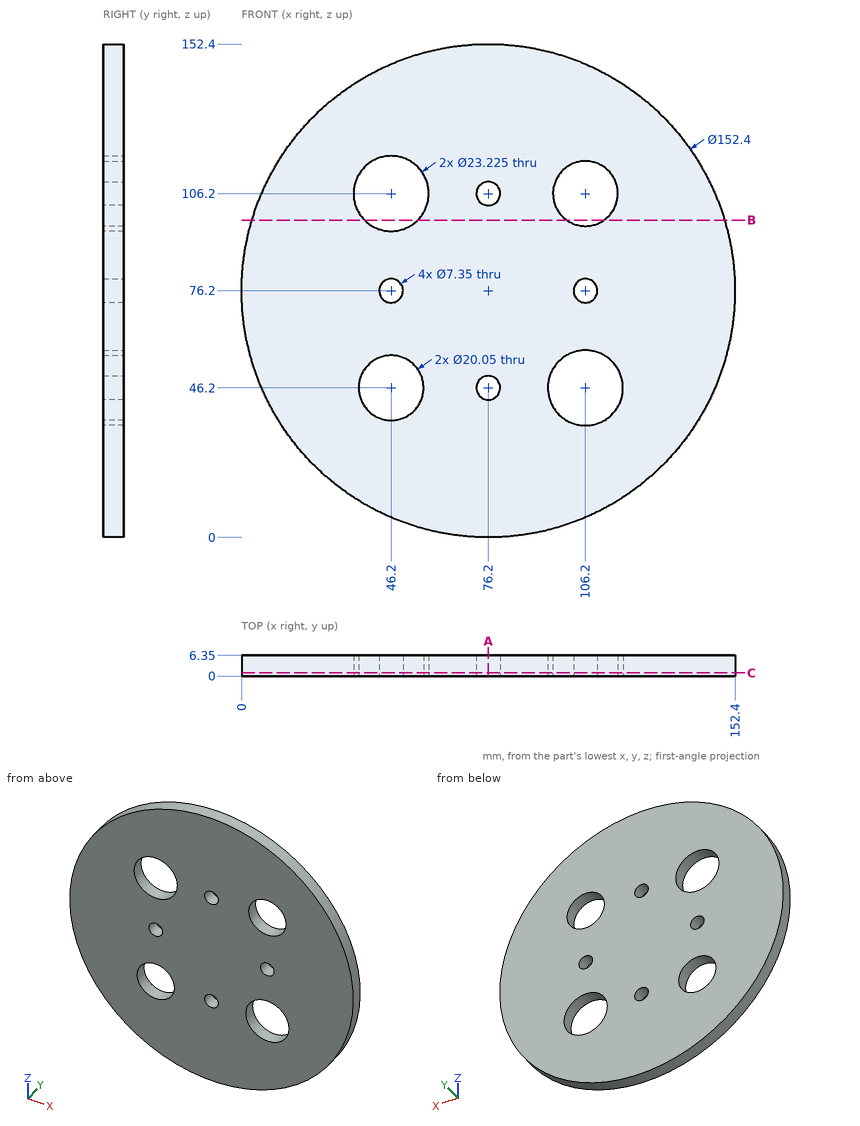
Here's the drawing with two shaded views (mm, measured from the low corner). I have some questions. Give positions to 0.01 mm unless a question says otherwise; leave off trailing zeros. Order: outer loops, then holes, each group sorted by start corner. A loop starts at its lowest first (then second) coordinate and runs counter-clockwise, first axis right, second up. Notation, with made-up numbers: (26.5, 56) -> (39.5, 56) arc R23 cw to (39.5, 75) -> close; hole circle Ø3 at (-24.75, 8.5). An arc over 180 degrees is marked (long way). One line per item, written item: value. Start each with the question number.
1. Imagine slicing it at C-C, the plane y = 1. Count the separate pieces of the cut face and the enclosed holes in it, plus the area to 3 significant figures.
2. Imagine slicing it at B-B, the plane z = 98. List the corners of the cut face in (x, y) for me, plus the area to 3 significant figures.
3. Imagine slicing it at A-A, the plane x = 76.2. List the corners of the cut face in (y, z) for me (3 decimals), plus the area to 3 significant figures.
4. Will these pins go through, and if not, where does the flat tip stop? pin 1 Ø2 at (y, z) = (4, 122) entering from -X; pin 2 Ø6.5 at (x, z) = (106.2, 76.2) entering from -Y.
5. I need wall thicknesses on probe 1 along X at (y, z) = (2, 76.2) (3 decimals); probe 2 along Z at (x, y) = (43.5, 2.75); probe 3 along Z at (x, y) = (46.2, 1.75) (1 decimal). Which ranges of each line are inside material? Lowest first, please. Write a range as from..to.
Values follow:
1. separate pieces: 1
1. enclosed holes: 8
1. area: 16,600 mm2
2. outline: (3.18, 0) -> (37.98, 0) -> (37.98, 6.35) -> (3.18, 6.35) -> close; (54.42, 0) -> (100.43, 0) -> (100.43, 6.35) -> (54.42, 6.35) -> close; (111.97, 0) -> (149.22, 0) -> (149.22, 6.35) -> (111.97, 6.35) -> close
2. area: 750 mm2
3. outline: (0, 0) -> (6.35, 0) -> (6.35, 42.525) -> (0, 42.525) -> close; (0, 49.875) -> (6.35, 49.875) -> (6.35, 102.525) -> (0, 102.525) -> close; (0, 109.875) -> (6.35, 109.875) -> (6.35, 152.4) -> (0, 152.4) -> close
3. area: 874 mm2
4. pin 1: stops at x = 14.56
4. pin 2: passes through
5. probe 1: x = 0..42.525, 49.875..102.525, 109.875..152.4
5. probe 2: z = 7.37..36.55, 55.85..73.71, 78.69..94.91, 117.49..145.03
5. probe 3: z = 6.2..36.2, 56.2..72.5, 79.9..94.6, 117.8..146.2
